Could you check a few things on this model? Use its own coordinates, in mm. A direction names the side the tool comes from. Coordinates: 2 decimals unless noted, no trailing zeros. Loops run counter-clockwise (first coordinate to the right, second up) from the corner with the lowest first, then second, coordinate; pieces in that order, holes last. Notation, with made-up numbers: (67, 25.5) -> (97, 25.5) arc R28 cw to (97, 44.5) -> close; hole circle Ø11 at (0, 47.25). An arc over 180 degrees is marked (long way). One line per question, with ' | ' between items.
```python
from build123d import *

# Parameters (mm, degrees)
BOSS_EXTRUDE1_DEPTH      = 70
BOSS_EXTRUDE1_DEPTH_BACK = 20
SKETCH1_R                = 120
SKETCH1_R_2              = 105
SKETCH2_R                = 105
SKETCH2_R_2              = 75
BOSS_EXTRUDE2_DEPTH      = 6
SKETCH3_R                = 120
SKETCH3_R_2              = 115
CUT_EXTRUDE1_DEPTH       = 193.093727123
SKETCH4_R                = 120
SKETCH4_R_2              = 110
CUT_EXTRUDE2_DEPTH       = 186.876302954


with BuildPart() as part:
    # Sketch1 → Boss-Extrude1 (new, two sides: drawn at the far end of the back side and taken through both)
    with BuildSketch(Plane(origin=(0, 0, 0), x_dir=(1, 0, 0), z_dir=(0, 1, 0)).offset(-BOSS_EXTRUDE1_DEPTH_BACK)):
        with Locations(Location((0, 0, 0), (0, 0, 270))):
            Circle(SKETCH1_R)
        with Locations(Location((0, 0, 0), (0, 0, 270))):
            Circle(SKETCH1_R_2, mode=Mode.SUBTRACT)
    extrude(amount=BOSS_EXTRUDE1_DEPTH + BOSS_EXTRUDE1_DEPTH_BACK)

    # Sketch2 → Boss-Extrude2 (add)
    with BuildSketch(Plane(origin=(0, 0, 0), x_dir=(1, 0, 0), z_dir=(0, 1, 0))):
        with Locations(Location((0, 0, 0), (0, 0, 270))):
            Circle(SKETCH2_R)
        with Locations(Location((0, 0, 0), (0, 0, 270))):
            Circle(SKETCH2_R_2, mode=Mode.SUBTRACT)
    extrude(amount=-BOSS_EXTRUDE2_DEPTH)

    # Sketch3 → Cut-Extrude1 (cut, through all)
    with BuildSketch(Plane(origin=(0, 70, 0), x_dir=(1, 0, 0), z_dir=(0, 1, 0))):
        Circle(SKETCH3_R)
        with Locations(Location((0, 0, 0), (0, 0, 270))):
            Circle(SKETCH3_R_2, mode=Mode.SUBTRACT)
    extrude(amount=-CUT_EXTRUDE1_DEPTH, mode=Mode.SUBTRACT)

    # Sketch4 → Cut-Extrude2 (cut, through all)
    with BuildSketch(Plane(origin=(0, 70, 0), x_dir=(1, 0, 0), z_dir=(0, 1, 0))):
        Circle(SKETCH4_R)
        with Locations(Location((0, 0, 0), (0, 0, 270))):
            Circle(SKETCH4_R_2, mode=Mode.SUBTRACT)
    extrude(amount=-CUT_EXTRUDE2_DEPTH, mode=Mode.SUBTRACT)


solid = part.part
```
Q1. For pin 1 (12 mm diameter, centred on y = 27.5, z = 85.5, fed in from -X); pin 2 (8 mm diameter, centred on x = 50.5, y = 3, fed in from +Z); pin 3 (3 mm diameter, centred on y = 57.5, z = -20.5, fed in from -X), each with a flat end and sliding along its axis, tell me the tip position at first contact or that it passes through.
Values follow:
pin 1: stops at x = -76.02 | pin 2: stops at z = 99.69 | pin 3: stops at x = -108.35
Q2. Please list where these lines run through material, in increasing order: L1, parallel to X at y = 45.5, z = 0; L2, parallel to X at y = -2, z = 0; L3, parallel to Z at x = -79.5, y = 9. Write a range as [from, to].
Values follow:
L1: x = [-110, -105], [105, 110] | L2: x = [-110, -75], [75, 110] | L3: z = [-76.02, -68.59], [68.59, 76.02]
Q3. Imagine slicing it at A-A on z = 0. Write out the boundary of the cut face in (x, y).
Values follow:
outline: (-110, -20) -> (-105, -20) -> (-105, -6) -> (-75, -6) -> (-75, 0) -> (-105, 0) -> (-105, 70) -> (-110, 70) -> close; (75, -6) -> (105, -6) -> (105, -20) -> (110, -20) -> (110, 70) -> (105, 70) -> (105, 0) -> (75, 0) -> close
Q4. For faces 4 (the face through (31.54, -13.1, 100.15)), 5 (the face through (31.54, 34.51, 100.15)), 6 (the face through (-40.2, 70, 97.3)), which set-ups out of +Z, -Z, +X, -X, +Y, -Y let a thin tool reach every point of the face, with its end or its side?
Values follow:
face 4: -Y | face 5: +Y | face 6: +Z, -Z, +X, -X, +Y
Q5. Imagine slicing it at D-D on z = 88. Write out the boundary of the cut face in (x, y), plus the area to 3 significant figures.
Values follow:
outline: (-66, -20) -> (-57.28, -20) -> (-57.28, -6) -> (57.28, -6) -> (57.28, -20) -> (66, -20) -> (66, 70) -> (57.28, 70) -> (57.28, 0) -> (-57.28, 0) -> (-57.28, 70) -> (-66, 70) -> close | area: 2,260 mm2
Q6. Imagine slicing it at C-C on y = 59.5. Write out the boundary of the cut face in (x, z).
Values follow:
outline: circle Ø220 at (0, 0); hole circle Ø210 at (0, 0)
Q7. We'd pull the mould along Z, two halves only. Please class faces 1 (the face through (-97.59, 25.63, 50.76)), 2 (the face through (25, 0, -71)), 3 (the face through (-40.2, -20, 97.3)): released by +Z, released by -Z, zero draft, split by the parting line, or undercut.
Values follow:
face 1: split by the parting line | face 2: undercut | face 3: zero draft
Q8. Imagine slicing it at B-B on x = 0. Write out the boundary of the cut face in (y, z).
Values follow:
outline: (-20, -110) -> (70, -110) -> (70, -105) -> (0, -105) -> (0, -75) -> (-6, -75) -> (-6, -105) -> (-20, -105) -> close; (-20, 105) -> (-6, 105) -> (-6, 75) -> (0, 75) -> (0, 105) -> (70, 105) -> (70, 110) -> (-20, 110) -> close
